Model file for the job. Use its own axes, mm. Round coordinates to 2 decimals unless told otherwise and drop trailing zeros. Order: outer loops, then holes, each group sorted by start corner. A loop starts at its lowest first (then second) coordinate and runs counter-clockwise, first axis right, second up. Notation, with made-up numbers: M 75.5,49 L 89.5,49 A17 ccw 89.5,59 Z; hole C 29,54 d9. An arc over 180 degrees is marked long. Return JSON: item names as keys, results as strings. Group by question number.
Item 1: Slice it at A-A on x = -96. Write the cut outline in (y, z), then the cut area to 3 significant figures.
Item 2: Slice it at B-B on y = 53. Write the cut outline in (x, z).
Item 3: Probe line 1 along Y through (x, z) = (-142.5, 2.45); line 2 along Y through (x, z) = (-7, 3.15); line 3 along X through (y, z) = (53.5, 0.85). List the from-to ranges inside material, lowest first.
Item 4: Slice it at C-C on y = 78.49. Write the cut outline in (x, z), then the cut area to 3 significant figures.
Item 5: Slice it at D-D on y = 41.5. Write the cut outline in (x, z), then the cut area to 3 significant figures.
from build123d import *

# Parameters (mm, degrees)
SKETCH_1_W           = 110
SKETCH_1_H           = 150
EXTRUDE_1_DEPTH      = 4
HOLE_WIZARD_M4_1_D   = 4.8
HOLE_WIZARD_M3_1_D   = 3.2
SKETCH_6_OUTSIDE_W   = 189.21
SKETCH_6_OUTSIDE_H   = 149.21
SKETCH_6_OUTSIDE_W_2 = 150
SKETCH_6_OUTSIDE_H_2 = 110
CUT_EXTRUDE_1_DEPTH  = 5
FILLET_3_R           = 5
FILLET_1_R           = 7.5


with BuildPart() as part:
    # ｽｹｯﾁ1 → ﾎﾞｽ - 押し出し1 (new body)
    with BuildSketch(Plane(origin=(0, 0, 0), x_dir=(0, 1, 0), z_dir=(0, 0, 1))):
        with Locations((55, 75)):
            Rectangle(SKETCH_1_W, SKETCH_1_H)
    extrude(amount=EXTRUDE_1_DEPTH)

    # M4 すきま穴1 (through all)
    with Locations(Plane.XY.offset(4)):
        with Locations((-142.5, 102.5), (-142.5, 7.5), (-7.5, 102.5), (-7.5, 7.5)):
            Hole(HOLE_WIZARD_M4_1_D / 2)

    # M3 すきま穴1 (through all)
    with Locations(Plane.XY.offset(4)):
        with Locations((-110, 31.5), (-33.8, 78.49)):
            Hole(HOLE_WIZARD_M3_1_D / 2)

    # ｽｹｯﾁ6 outside → ｶｯﾄ - 押し出し1 (cut, through all)
    with BuildSketch(Plane.XY.offset(4)):
        with Locations((-75, 55)):
            Rectangle(SKETCH_6_OUTSIDE_W, SKETCH_6_OUTSIDE_H)
        with Locations((-75, 55)):
            Rectangle(SKETCH_6_OUTSIDE_W_2, SKETCH_6_OUTSIDE_H_2, mode=Mode.SUBTRACT)
        Polygon((-126.666666667, 10), (-23.333333333, 10), (-75, 48.75), align=None)
        with BuildLine():
            Line((-135, 16.25), (-135, 93.75))
            Line((-135, 93.75), (-83.333333333, 55))
            Line((-83.333333333, 55), (-107.434720268, 36.923959799))
            ThreePointArc((-107.434720268, 36.923959799), (-113.6, 36.3), (-115.925279732, 30.556040201))
            Line((-115.925279732, 30.556040201), (-135, 16.25))
        make_face()
        Polygon((-126.666666667, 100), (-23.333333333, 100), (-75, 61.25), align=None)
        with BuildLine():
            Line((-15, 16.25), (-15, 93.75))
            Line((-15, 93.75), (-29.614559787, 82.78908016))
            ThreePointArc((-29.614559787, 82.78908016), (-30.2, 73.69), (-39.099040213, 75.67571984))
            Line((-39.099040213, 75.67571984), (-66.666666667, 55))
            Line((-66.666666667, 55), (-15, 16.25))
        make_face()
    extrude(amount=-CUT_EXTRUDE_1_DEPTH, mode=Mode.SUBTRACT)

    # ﾌｨﾚｯﾄ3
    fillet_3_edges = [part.edges().sort_by_distance(p)[0] for p in [
        (-75, 48.75, 2),
        (-23.333333333, 10, 2),
        (-126.666666667, 10, 2),
        (-135, 93.75, 2),
        (-83.333333333, 55, 2),
        (-107.434720268, 36.923959799, 2),
        (-115.925279732, 30.556040201, 2),
        (-135, 16.25, 2),
        (-15, 16.25, 2),
        (-66.666666667, 55, 2),
        (-39.099040213, 75.67571984, 2),
        (-29.614559787, 82.78908016, 2),
        (-15, 93.75, 2),
        (-75, 61.25, 2),
        (-126.666666667, 100, 2),
        (-23.333333333, 100, 2),
    ]]
    fillet(fillet_3_edges, radius=FILLET_3_R)

    # ﾌｨﾚｯﾄ1
    fillet_1_edges = [part.edges().sort_by_distance(p)[0] for p in [
        (-150, 0, 2),
        (-150, 110, 2),
        (0, 110, 2),
        (0, 0, 2),
    ]]
    fillet(fillet_1_edges, radius=FILLET_1_R)


solid = part.part
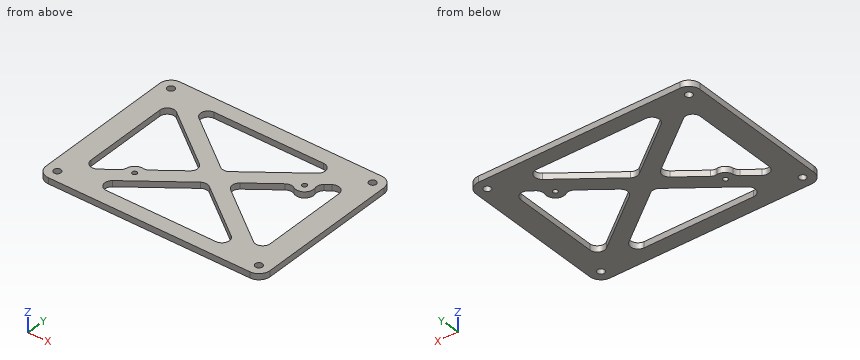
Output values:
{
 "1": {"outline": "M 0,0 L 10,0 L 10,4 L 0,4 Z; M 33,0 L 45.5,0 L 45.5,4 L 33,4 Z; M 64.5,0 L 77,0 L 77,4 L 64.5,4 Z; M 100,0 L 110,0 L 110,4 L 100,4 Z", "area": "180 mm²"},
 "2": {"outline": "M -150,0 L -135,0 L -135,4 L -150,4 Z; M -87.08,0 L -62.92,0 L -62.92,4 L -87.08,4 Z; M -15,0 L 0,0 L 0,4 L -15,4 Z"},
 "3": {"line 1": "0 to 5.1, 9.9 to 100.1, 104.9 to 110", "line 2": "0.02 to 5.15, 9.85 to 100.15, 104.85 to 109.98", "line 3": "-150 to -135, -86.9 to -63.1, -15 to 0"},
 "4": {"outline": "M -150,0 L -135,0 L -135,4 L -150,4 Z; M -114.65,0 L -97.99,0 L -97.99,4 L -114.65,4 Z; M -52.01,0 L -35.4,0 L -35.4,4 L -52.01,4 Z; M -32.2,0 L -27.8,0 L -27.8,4 L -32.2,4 Z; M -15,0 L 0,0 L 0,4 L -15,4 Z", "area": "271 mm²"},
 "5": {"outline": "M -150,0 L -135,0 L -135,4 L -150,4 Z; M -101.33,0 L -84.67,0 L -84.67,4 L -101.33,4 Z; M -65.33,0 L -48.67,0 L -48.67,4 L -65.33,4 Z; M -15,0 L 0,0 L 0,4 L -15,4 Z", "area": "253 mm²"}
}
